```python
from build123d import *

# Parameters (mm, degrees)
BOSS_EXTRUDE1_DEPTH = 10
CUT_EXTRUDE1_DEPTH  = 10
FILLET1_R           = 2


with BuildPart() as part:
    # Sketch1 → Boss-Extrude1 (new body)
    with BuildSketch(Plane.XY):
        with BuildLine():
            Line((-0.39684881, -4.080748831), (-0.39684881, -14.87796999))
            Line((-0.39684881, -14.87796999), (-3.39684881, -14.87796999))
            Line((-3.39684881, -14.87796999), (-3.39684881, -4.87796999))
            ThreePointArc((-3.39684881, -4.87796999), (0, 5.944171352), (3.39684881, -4.87796999))
            Line((3.39684881, -4.87796999), (3.39684881, -14.87796999))
            Line((3.39684881, -14.87796999), (0.39684881, -14.87796999))
            Line((0.39684881, -14.87796999), (0.39684881, -4.080748831))
            ThreePointArc((0.39684881, -4.080748831), (0, 4.1), (-0.39684881, -4.080748831))
        make_face()
    extrude(amount=BOSS_EXTRUDE1_DEPTH)

    # Sketch2 → Cut-Extrude1 (cut)
    with BuildSketch(Plane(origin=(3.39684881, 0, 0), x_dir=(0, 0, -1), z_dir=(1, 0, 0))):
        with BuildLine():
            ThreePointArc((-3.12616703, -8.004137019), (-6.87383297, -8.004137019), (-6.87383297, -11.75180296))
            Line((-6.87383297, -11.75180296), (-3.12616703, -8.004137019))
        make_face()
        with BuildLine():
            Line((-3.12616703, -8.004137019), (-6.87383297, -11.75180296))
            ThreePointArc((-6.87383297, -11.75180296), (-3.985888904, -12.326250751), (-2.35, -9.87796999))
            ThreePointArc((-2.35, -9.87796999), (-2.551719239, -8.863858894), (-3.12616703, -8.004137019))
        make_face()
    extrude(amount=-CUT_EXTRUDE1_DEPTH, mode=Mode.SUBTRACT)

    # Fillet1
    fillet1_edges = [part.edges().sort_by_distance(p)[0] for p in [
        (1.89684881, -14.87796999, 0),
        (1.89684881, -14.87796999, 10),
        (-1.89684881, -14.87796999, 10),
        (-1.89684881, -14.87796999, 0),
    ]]
    fillet(fillet1_edges, radius=FILLET1_R)


solid = part.part
```
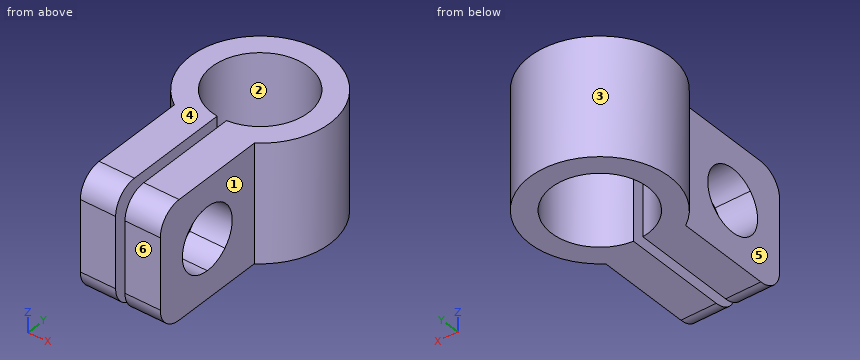
For this review, take the finished solid that the model builds, in its own axes (mm). Face numbers are marked on the shaded views. A direction names the side the tool comes from. Coordinates: 2 decimals unless noted, no trailing zeros. Write each loop counter-clockwise with the first axis right and the second up, starting at its lowest first coordinate (ties: lowest second). Pieces come first, ordered by that corner, then holes.
(1) Wall thickness on probe 1 along X at (y, z) = (-9.5, 8); probe 2 along X at (y, z) = (0, 4.5); probe 3 along Y at (x, z) = (-0.75, 5.5): over which ranges is each line inside the solid? List them lowest first.
(2) Add section D-D on y = -7.5. Give the boundary of the cut face in (x, z).
(3) Tool access review of the marked faces 5 and 6: name each direction out of +Z, -Z, +X, -X, +Y, -Y from which nothing blocks a thin tool from reaching the whole face with its end or side.
(4) Add section C-C on z = 5. Give the boundary of the cut face in (x, y).
(5) For pin 1 Ø5 at (y, z) = (-10.5, 2.5) entering from +X; pin 2 Ø3 at (y, z) = (-9, 2.5) entering from -X, all flat-tipped, find the tip position at first contact; note any pin that passes through.
(6) The part is to be moulded in two halves that separate along X. For the marked faces 1, 2, 3 and 4, say which applies: +X half, -X half, draft (parallel to the pull), parting line (faces both ways), or undercut.
(7) Add section B-B on x = -1.25. Give the boundary of the cut face in (y, z).
(8) Add section A-A on y = 0. Give the boundary of the cut face in (x, z).
Answer sheet:
1. probe 1: x = -3.4 to -0.4, 0.4 to 3.4
1. probe 2: x = -5.94 to -4.1, 4.1 to 5.94
1. probe 3: y = -14.88 to -12.48, -7.28 to -4.03, 4.03 to 5.9
2. outline: (-3.4, 0) - (-0.4, 0) - (-0.4, 3.83) - (-3.4, 3.83) - close; (-3.4, 6.17) - (-0.4, 6.17) - (-0.4, 10) - (-3.4, 10) - close; (0.4, 0) - (3.4, 0) - (3.4, 3.83) - (0.4, 3.83) - close; (0.4, 6.17) - (3.4, 6.17) - (3.4, 10) - (0.4, 10) - close
3. face 5: +Z, -Z, -X, -Y
3. face 6: +Z, -Z, +X, -X, -Y
4. outline: (-3.4, -14.88) - (-0.4, -14.88) - (-0.4, -12.53) - (-3.4, -12.53) - close; (-3.4, -7.23) - (-0.4, -7.23) - (-0.4, -4.08) arc R4.1 cw (long way) to (0.4, -4.08) - (0.4, -7.23) - (3.4, -7.23) - (3.4, -4.88) arc R5.94 ccw (long way) to (-3.4, -4.88) - close; (0.4, -14.88) - (3.4, -14.88) - (3.4, -12.53) - (0.4, -12.53) - close
5. pin 1: stops at x = 3.4
5. pin 2: stops at x = -3.4
6. face 1: +X half
6. face 2: undercut
6. face 3: parting line
6. face 4: draft
7. outline: (-14.88, 2) arc R2 ccw to (-12.88, 0) - (-3.9, 0) - (-3.9, 10) - (-12.88, 10) arc R2 ccw to (-14.88, 8) - close; (3.9, 0) - (5.81, 0) - (5.81, 10) - (3.9, 10) - close; hole circle Ø5.3 at (-9.88, 5)
8. outline: (-5.94, 0) - (-4.1, 0) - (-4.1, 10) - (-5.94, 10) - close; (4.1, 0) - (5.94, 0) - (5.94, 10) - (4.1, 10) - close
